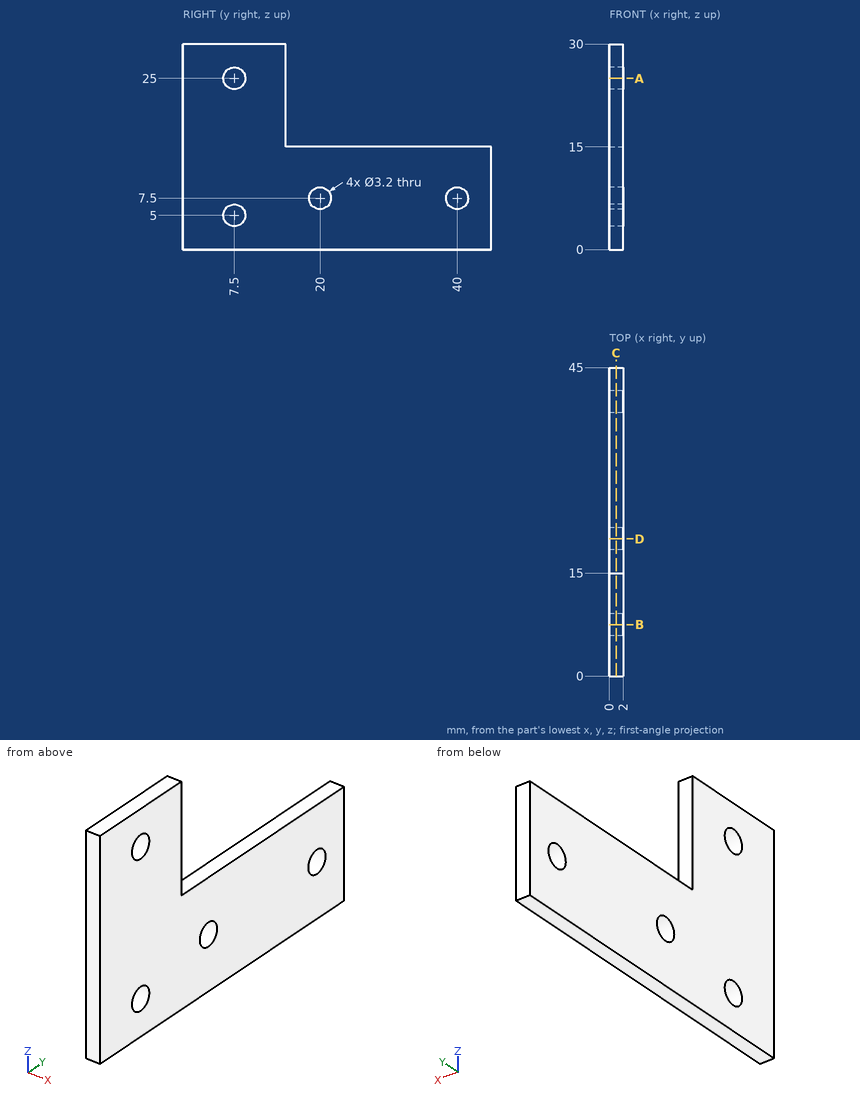
Study the drawing (mm; zero at the part's minimum x, y, z) and answer. Give positions to 0.01 mm unless a question says otherwise; leave off trailing zeros. Write each loop counter-clockwise with the first axis right and the second up, starting at its lowest first coordinate (ties: lowest second). Pieces come first, ordered by that corner, then holes. Notation, with made-up numbers: (-32.75, 88.25) -> (26.25, 88.25) arc R22 ccw to (26.25, 123.25) -> close; hole circle Ø2 at (-29.5, 68.5). An arc over 180 degrees is marked (long way). Answer in a Markdown table with one row per item.
1) Section C-C on x = 1 is taken. Give the vertices of the cut face in (y, z), plus the area to 3 significant figures.
Results list:
| item | result |
|---|---|
| outline | (0, 0) -> (45, 0) -> (45, 15) -> (15, 15) -> (15, 30) -> (0, 30) -> close; hole circle Ø3.2 at (7.5, 5); hole circle Ø3.2 at (7.5, 25); hole circle Ø3.2 at (20, 7.5); hole circle Ø3.2 at (40, 7.5) |
| area | 868 mm^2 |
2) Section B-B on y = 7.5 is taken. Give the vertices of the cut face in (x, z), plus the area to 3 significant figures.
Results list:
| item | result |
|---|---|
| outline | (0, 0) -> (2, 0) -> (2, 3.4) -> (0, 3.4) -> close; (0, 6.6) -> (2, 6.6) -> (2, 23.4) -> (0, 23.4) -> close; (0, 26.6) -> (2, 26.6) -> (2, 30) -> (0, 30) -> close |
| area | 47.2 mm^2 |
3) Section A-A on z = 25 is taken. Give the vertices of the cut face in (x, y).
Results list:
| item | result |
|---|---|
| outline | (0, 0) -> (2, 0) -> (2, 5.9) -> (0, 5.9) -> close; (0, 9.1) -> (2, 9.1) -> (2, 15) -> (0, 15) -> close |
4) This flat-tipped pin is pushed along its axis until it touches: pin 1 Ø1 at (x, y) = (1, 27) entering from +Z. Where does it stop, or does it pass through?
Results list:
| item | result |
|---|---|
| pin 1 | z = 15 |
5) Straight lines are drawn through the part: line 1 (Z direction, x = 1.65, y = 7.5); line 2 (Y direction, x = 0.4, z = 7.5); line 3 (Y direction, x = 1.2, z = 5). For each, find the intervals that lie inside material, in ascending order. Write a range as [from, to].
Results list:
| item | result |
|---|---|
| line 1 | [0, 3.4], [6.6, 23.4], [26.6, 30] |
| line 2 | [0, 18.4], [21.6, 38.4], [41.6, 45] |
| line 3 | [0, 5.9], [9.1, 45] |
